from build123d import *

# Parameters (mm, degrees)
SKETCH1_R           = 1.5
SKETCH1_R_2         = 6.35
SKETCH1_W           = 25.4
SKETCH1_H           = 5.08
SKETCH1_W_2         = 5.08
SKETCH1_H_2         = 25.4
BOSS_EXTRUDE1_DEPTH = 5.08


with BuildPart() as part:
    # Sketch1 → Boss-Extrude1 (new body)
    with BuildSketch(Plane.XY):
        with BuildLine():
            Line((-51.040787545, -12.415612204), (-51.040787545, -9.875612204))
            ThreePointArc((-51.040787545, -9.875612204), (-48.808941218, -4.487458531), (-43.420787545, -2.255612204))
            Line((-43.420787545, -2.255612204), (119.139212455, -2.255612204))
            ThreePointArc((119.139212455, -2.255612204), (124.527366128, -4.487458531), (126.759212455, -9.875612204))
            Line((126.759212455, -9.875612204), (126.759212455, -12.415612204))
            ThreePointArc((126.759212455, -12.415612204), (127.503161231, -14.211663428), (129.299212455, -14.955612204))
            Line((129.299212455, -14.955612204), (136.919212455, -14.955612204))
            ThreePointArc((136.919212455, -14.955612204), (138.715263679, -14.211663428), (139.459212455, -12.415612204))
            Line((139.459212455, -12.415612204), (139.459212455, 63.784387796))
            ThreePointArc((139.459212455, 63.784387796), (132.763673473, 79.948848814), (116.599212455, 86.644387796))
            Line((116.599212455, 86.644387796), (98.187659058, 86.644387796))
            Line((98.187659058, 86.644387796), (66.292302759, 118.539744095))
            ThreePointArc((66.292302759, 118.539744095), (64.089891606, 121.835885319), (63.316507656, 125.723948992))
            Line((63.316507656, 125.723948992), (63.316507656, 295.368236906))
            ThreePointArc((63.316507656, 295.368236906), (60.340712553, 302.552441803), (53.156507656, 305.528236906))
            Line((53.156507656, 305.528236906), (27.774726543, 305.528236906))
            ThreePointArc((27.774726543, 305.528236906), (20.590521646, 302.552441803), (17.614726543, 295.368236906))
            Line((17.614726543, 295.368236906), (17.614726543, 125.723948992))
            ThreePointArc((17.614726543, 125.723948992), (16.841342593, 121.835885319), (14.63893144, 118.539744095))
            Line((14.63893144, 118.539744095), (-17.256424859, 86.644387796))
            Line((-17.256424859, 86.644387796), (-40.880787545, 86.644387796))
            ThreePointArc((-40.880787545, 86.644387796), (-57.045248563, 79.948848814), (-63.740787545, 63.784387796))
            Line((-63.740787545, 63.784387796), (-63.740787545, -12.415612204))
            ThreePointArc((-63.740787545, -12.415612204), (-62.996838769, -14.211663428), (-61.200787545, -14.955612204))
            Line((-61.200787545, -14.955612204), (-53.580787545, -14.955612204))
            ThreePointArc((-53.580787545, -14.955612204), (-51.784736321, -14.211663428), (-51.040787545, -12.415612204))
        make_face()
        with Locations((37.859212455, 50.082420202)):
            Circle(SKETCH1_R, mode=Mode.SUBTRACT)
        with Locations((78.378833182, 8.65637608)):
            Circle(SKETCH1_R, mode=Mode.SUBTRACT)
        with Locations(Location((-2.660408273, 8.65637608, 0), (0, 0, 180))):
            Circle(SKETCH1_R, mode=Mode.SUBTRACT)
        with Locations((49.670678041, 298.310354304)):
            Circle(SKETCH1_R, mode=Mode.SUBTRACT)
        with Locations((49.670678041, 262.606350585)):
            Circle(SKETCH1_R, mode=Mode.SUBTRACT)
        with Locations((49.670678041, 280.294601083)):
            Circle(SKETCH1_R_2, mode=Mode.SUBTRACT)
        with Locations((37.859212455, 202.482420202)):
            Circle(SKETCH1_R, mode=Mode.SUBTRACT)
        with Locations((103.536086771, 8.65637608)):
            Rectangle(SKETCH1_W, SKETCH1_H, mode=Mode.SUBTRACT)
        with Locations((-27.817661861, 8.65637608)):
            Rectangle(SKETCH1_W, SKETCH1_H, mode=Mode.SUBTRACT)
        with Locations((37.859212455, 66.389058861)):
            Rectangle(SKETCH1_W_2, SKETCH1_H_2, mode=Mode.SUBTRACT)
        with Locations((37.859212455, 218.789058861)):
            Rectangle(SKETCH1_W_2, SKETCH1_H_2, mode=Mode.SUBTRACT)
    extrude(amount=BOSS_EXTRUDE1_DEPTH)


solid = part.part
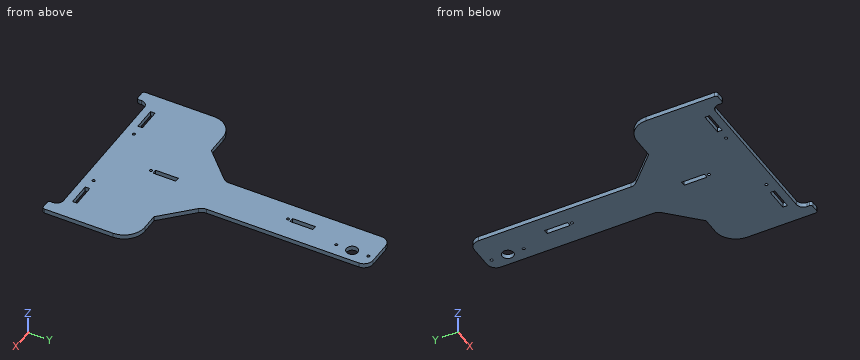
CAD build for the part. Positions are in the model's coordinates, mm. Coordinates: 2 decimals unless noted, no trailing zeros. Write each loop counter-clockwise with the first axis right and the second up, starting at its lowest first coordinate (ties: lowest second). Pieces come first, ordered by that corner, then holes. Notation, with made-up numbers: M -12.5,51 L 31.5,51 A13 ccw 31.5,58 Z; hole C -18.5,64.5 d1. An arc over 180 degrees is marked long. Return JSON: item names as keys, results as strings.
Item 1: Probe line 1 (X direction, y = 218, z = 2.4); line 2 (Y direction, x = -20, z = 3.4); line 3 (X direction, y = 273, z = 4.3). List the from-to ranges inside material, lowest first. Write a range as from..to.
Findings below:
{"line 1": "x = 17.61..35.32, 40.4..63.32", "line 2": "y = -2.26..6.12, 11.2..86.64", "line 3": "x = 17.61..63.32"}
Item 2: Drop flat-ended pins along their axis: pin 1 Ø3 at (x, z) = (106, 3) entering from -Y; pin 2 Ø1.5 at (x, z) = (-29, 3) entering from +Y; pin 3 Ø1.5 at (y, z) = (192.5, 3.5) entering from +X. Give the stop position or say it passes through.
Findings below:
{"pin 1": "stops at y = -2.26", "pin 2": "stops at y = 86.64", "pin 3": "stops at x = 63.32"}
Item 3: Slice it at B-B, the plane y = 220. Write the cut outline in (x, z), and give its area (3 significant figures).
Findings below:
{"outline": "M 17.61,0 L 35.32,0 L 35.32,5.08 L 17.61,5.08 Z; M 40.4,0 L 63.32,0 L 63.32,5.08 L 40.4,5.08 Z", "area": "206 mm2"}
Item 4: Slice it at A-A, the plane x = -22. Write the cut outline in (y, z).
Findings below:
{"outline": "M -2.26,0 L 6.12,0 L 6.12,5.08 L -2.26,5.08 Z; M 11.2,0 L 86.64,0 L 86.64,5.08 L 11.2,5.08 Z"}
Item 5: Slice it at D-D, the plane y = 163. Write the cut outline in (x, z), and give its area (3 significant figures).
Findings below:
{"outline": "M 17.61,0 L 63.32,0 L 63.32,5.08 L 17.61,5.08 Z", "area": "232 mm2"}
Item 6: Slice it at C-C, the plane z = 2. State how many separate pieces and enclosed holes the cut face has, and give its area (3 significant figures).
Findings below:
{"separate pieces": "1", "enclosed holes": "11", "area": "28,700 mm2"}
